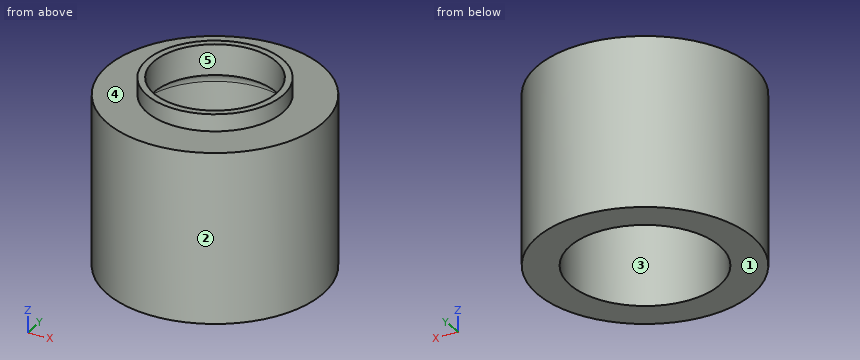
```python
from build123d import *

# Parameters (mm, degrees)
F0_R     = 15.875
F0_R_2   = 9
F1_DEPTH = 25
F2_R     = 10
F2_R_2   = 9
F3_DEPTH = 2.5
F4_R     = 11
F4_R_2   = 9
F5_DEPTH = 23
F6_R     = 1.99999
F7_DEPTH = 2.5


# Not quite as in the source:
# - a fillet or chamfer is up to 0.001 mm smaller than in the source, because OpenCascade refuses the exact size


with BuildPart() as f1:
    # F0 (on Top) → F1 (new body)
    with BuildSketch(Plane.XY):
        Circle(F0_R)
        Circle(F0_R_2, mode=Mode.SUBTRACT)
    extrude(amount=F1_DEPTH)

    # F2 (on face) → F3 (join)
    with BuildSketch(Plane.XY.offset(25)):
        Circle(F2_R)
        Circle(F2_R_2, mode=Mode.SUBTRACT)
    extrude(amount=F3_DEPTH)

    # F4 (on face) → F5 (cut)
    with BuildSketch(Plane(origin=(0, 0, 0), x_dir=(1, 0, 0), z_dir=(0, 0, -1))):
        Circle(F4_R)
        Circle(F4_R_2, mode=Mode.SUBTRACT)
    extrude(amount=-F5_DEPTH, mode=Mode.SUBTRACT)

    # F6 (radius 2 in the source; OpenCascade refuses exactly that, so slightly less here)
    f6_edges = [f1.edges().sort_by_distance(p)[0] for p in [
        (-11, 0, 23),
    ]]
    fillet(f6_edges, radius=F6_R)

    # F2 (on face) → F7 (join)
    with BuildSketch(Plane.XY.offset(25)):
        Circle(F2_R)
        Circle(F2_R_2, mode=Mode.SUBTRACT)
    extrude(amount=F7_DEPTH)


solid = f1.part
```
Source: CAD feature listing. Evaluate the final solid. Frame: model axes, mm. Face numbers are marked on the shaded views. A direction names the side the tool comes from. Round coordinates to 2 decimals unless told otherwise and drop trailing zeros. Order: outer loops, then holes, each group sorted by start corner. A loop starts at its lowest first (then second) coordinate and runs counter-clockwise, first axis right, second up. Notation, with made-up numbers: (20, 49.25) -> (65, 49.25) arc R32 ccw to (65, 84.25) -> close; hole circle Ø8 at (59, -7.5). An arc over 180 degrees is marked (long way). Use CSV: the item, a comma, the result in double quotes.
(1) Section C-C on z = 11.75. Return the cut outline in (x, y) (3 decimals), and give its area (3 significant figures).
Report:
outline,"circle Ø31.75 at (0, 0); hole circle Ø22 at (0, 0)"
area,"412 mm^2"
(2) Access query for the marked faces 4 and 5. Directions: +Z, -Z, +X, -X, +Y, -Y. A direction counts if a zero-diameter tool reaches every point of the face in a straight line with its end or side. Return the directions, or none.
Report:
face 4,"+Z"
face 5,"+Z, -Z"
(3) First-contact query: pin 1 Ø14.5 at (x, y) = (3, 1) entering from -Z; pin 2 Ø3 at (x, z) = (-6, 3.5) entering from +Y; pin 3 Ø1 at (y, z) = (-5, 10.5) entering from -X; pin 4 Ø12 at (y, z) = (5, 16) entering from +X (3 decimals). Flat tips, straight axial feed; report the tip coordinate or a pass-through.
Report:
pin 1,"z = 22.42"
pin 2,"y = 15.22"
pin 3,"x = -15.22"
pin 4,"x = 15.875"
(4) Ray query, L1, parallel to Y at x = 0, z = 5.5 (3 decimals); L2, parallel to Y at x = 0, z = 26.35; L3, parallel to X at y = -5.5, z = 25.5. Return the intervals inside material, ascending.
Report:
L1,"-15.875 to -11, 11 to 15.875"
L2,"-10 to -9, 9 to 10"
L3,"-8.35 to -7.12, 7.12 to 8.35"
(5) Pull-direction query (Y, two-part tool) for the marked faces 1, 2 and 3; classes: +Y half, -Y half, draft (parallel to the pull), parting line (faces both ways), or undercut.
Report:
face 1,"draft"
face 2,"parting line"
face 3,"undercut"
